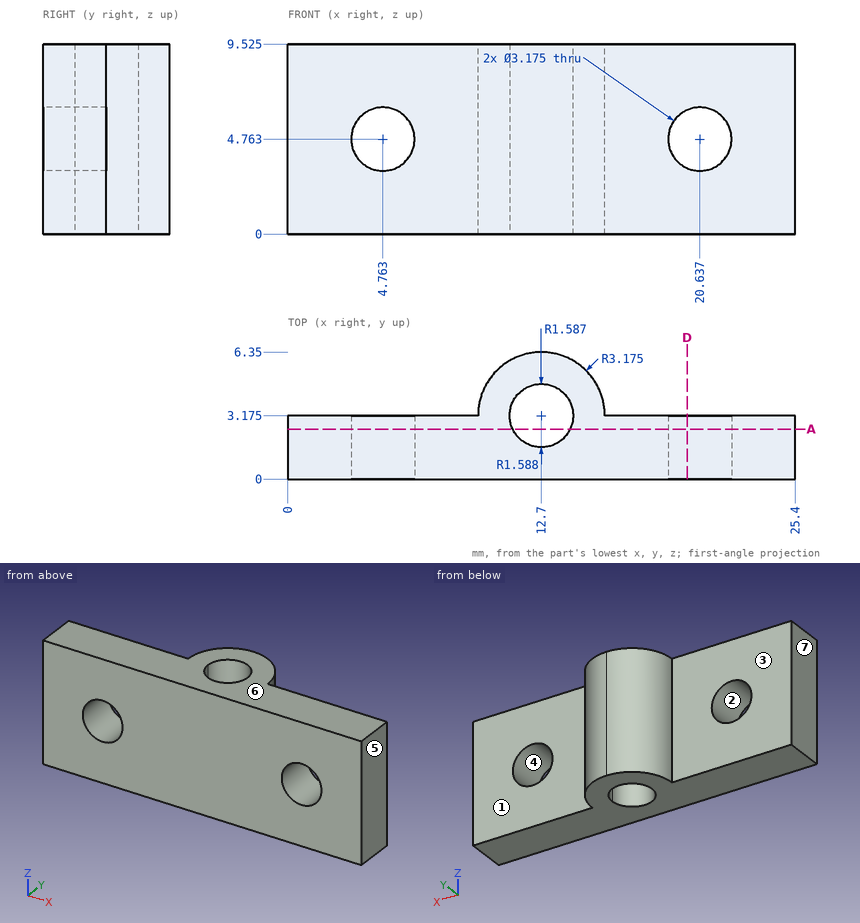
Design review of the part shown in the three views and the two pictorial views. Dimensions are in mm from the part's minimum x, y and z. A direction names the side the tool comes from. Round coordinates to 2 decimals unless told otherwise and drop trailing zeros. Order: outer loops, then holes, each group sorted by start corner. A loop starts at its lowest first (then second) coordinate and runs counter-clockwise, first axis right, second up.
Item 1: Add section A-A, the plane y = 2.5. Count the separate pieces of the cut face and the enclosed holes in it, and give its area (3 significant figures).
Working result:
separate pieces: 2
enclosed holes: 2
area: 199 mm2
Item 2: To check wall thickness, follow probe 1 along Y at (x, z) = (12, 6.25); probe 2 along X at (y, z) = (1.25, 4.25) (1 decimal); probe 3 along Y at (x, z) = (2.5, 8.25) (1 decimal). State the ranges of each line that lie inside material, in increasing order.
Working result:
probe 1: y = 0 to 1.75, 4.6 to 6.27
probe 2: x = 0 to 3.3, 6.3 to 19.1, 22.1 to 25.4
probe 3: y = 0 to 3.2
Item 3: Draft analysis for pull direction X (two halves, no side actions). For the marked faces 4, 5, 6 and 7, state which applies: released by +X, released by -X, zero draft, split by the parting line, or undercut.
Working result:
face 4: undercut
face 5: released by +X
face 6: zero draft
face 7: released by -X
Item 4: Add section D-D, the plane x = 20. State the section outline as (y, z) points (1 decimal), and give its area (3 significant figures).
Working result:
outline: (0, 0) - (3.2, 0) - (3.2, 3.3) - (0, 3.3) - close; (0, 6.2) - (3.2, 6.2) - (3.2, 9.5) - (0, 9.5) - close
area: 21.0 mm2
Item 5: Machinability: for the marked faces 1, 2 and 3, which of the approach directions +Z, -Z, +X, -X, +Y, -Y give a long, thin tool a straight path to every point of the face, cutting with its end or side? Answer none if there is none.
Working result:
face 1: +Z, -Z, +X, +Y
face 2: +Y, -Y
face 3: +Z, -Z, -X, +Y
Item 6: For pin 1 (2 mm diameter, centred on x = 5.5, z = 1.5, fed in from +Y) (1 decimal); pin 2 (1.5 mm diameter, centred on x = 5, y = 3.5, fed in from -Z); pin 3 (1 mm diameter, centred on y = 5.5, z = 4.5, fed in from -X); pin 4 (1.9 mm diameter, centred on x = 20.64, z = 4.76, fed in from -Y), all flat-tipped, find the tip position at first contact; note any pin that passes through.
Working result:
pin 1: stops at y = 3.2
pin 2: stops at z = 0
pin 3: stops at x = 10.1
pin 4: passes through
